from build123d import *

# Parameters (mm, degrees)
F0_W     = 317.5
F0_H     = 304.8
F1_DEPTH = 25.4
F2_W     = 317.5
F2_H     = 12.7
F3_DEPTH = 6.35
F4_W     = 317.5
F4_H     = 12.7
F5_DEPTH = 6.35
F8_DEPTH = 6.35
F9_DEPTH = 6.35


with BuildPart() as f1:
    # F0 (on Top) → F1 (new body)
    with BuildSketch(Plane.XY):
        Rectangle(F0_W, F0_H)
    extrude(amount=F1_DEPTH)

    # F2 (on face) → F3 (join)
    with BuildSketch(Plane(origin=(0, 152.4, 0), x_dir=(-1, 0, 0), z_dir=(0, 1, 0))):
        with Locations((0, 12.7)):
            Rectangle(F2_W, F2_H)
    extrude(amount=F3_DEPTH)

    # F4 (on face) → F5 (join)
    with BuildSketch(Plane.XZ.offset(152.4)):
        with Locations((0, 12.7)):
            Rectangle(F4_W, F4_H)
    extrude(amount=F5_DEPTH)

    # F7 (on face) → F8 (join)
    with BuildSketch(Plane(origin=(-158.75, 0, 0), x_dir=(0, -1, 0), z_dir=(-1, 0, 0))):
        Polygon((-152.4, 19.05), (-158.75, 19.05), (-158.75, 6.35), (-152.4, 6.35), (152.4, 6.35), (158.75, 6.35), (158.75, 19.05), (152.4, 19.05), align=None)
    extrude(amount=F8_DEPTH)

    # F6 (on face) → F9 (join)
    with BuildSketch(Plane.YZ.offset(158.75)):
        Polygon((-152.4, 19.05), (-158.75, 19.05), (-158.75, 6.35), (-152.4, 6.35), (152.4, 6.35), (158.75, 6.35), (158.75, 19.05), (152.4, 19.05), align=None)
    extrude(amount=F9_DEPTH)


solid = f1.part
The model under review builds one solid part; all positions refer to its coordinate system, in mm. Round coordinates to 2 decimals unless told otherwise and drop trailing zeros. Loops run counter-clockwise (first coordinate to the right, second up) from the corner with the lowest first, then second, coordinate; pieces in that order, holes last. Notation, with made-up numbers: (4.5, 61.5) -> (31.5, 61.5) arc R22 cw to (31.5, 81.5) -> close; hole circle Ø3 at (61.25, -22.75). An arc over 180 degrees is marked (long way). One line per question, with ' | ' between items. Start each with the question number.
Item 1: Add section B-B, the plane x = 55.5. Write out the cut boundary in (y, z).
Item 2: Wall thickness on line 1 along Y through (x, z) = (-120, 1.5); line 2 along X through (y, z) = (-17, 19.25): over which ranges is each line inside the solid? List them lowest first. Write a range as [from, to].
Item 3: For pin 1 (1.9 mm diameter, centred on x = 51.5, z = 3.5, fed in from -Y); pin 2 (5 mm diameter, centred on y = -31.5, z = 22.5, fed in from -X); pin 3 (3 mm diameter, centred on x = 67.5, z = 21.5, fed in from +Y), all flat-tipped, find the tip position at first contact; note any pin that passes through.
Item 4: Add section A-A, the plane y = 10. Write out the cut boundary in (x, z), then the cut area to 3 significant figures.
Return value:
1) outline: (-158.75, 6.35) -> (-152.4, 6.35) -> (-152.4, 0) -> (152.4, 0) -> (152.4, 6.35) -> (158.75, 6.35) -> (158.75, 19.05) -> (152.4, 19.05) -> (152.4, 25.4) -> (-152.4, 25.4) -> (-152.4, 19.05) -> (-158.75, 19.05) -> close
2) line 1: y = [-152.4, 152.4] | line 2: x = [-158.75, 158.75]
3) pin 1: stops at y = -152.4 | pin 2: stops at x = -158.75 | pin 3: stops at y = 152.4
4) outline: (-165.1, 6.35) -> (-158.75, 6.35) -> (-158.75, 0) -> (158.75, 0) -> (158.75, 6.35) -> (165.1, 6.35) -> (165.1, 19.05) -> (158.75, 19.05) -> (158.75, 25.4) -> (-158.75, 25.4) -> (-158.75, 19.05) -> (-165.1, 19.05) -> close | area: 8,230 mm2
